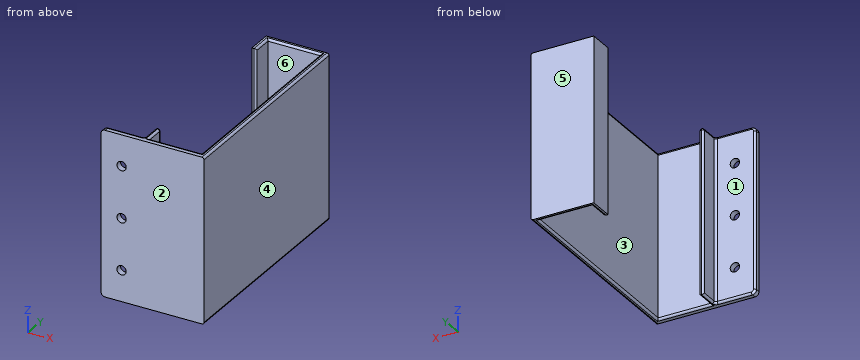
from build123d import *

# Parameters (mm, degrees)
SKETCH1_W           = 50
SKETCH1_H           = 80
BOSS_EXTRUDE1_DEPTH = 3
SKETCH2_R           = 2.25
CUT_EXTRUDE1_DEPTH  = 48.265209192
SKETCH3_W           = 2.8
SKETCH3_H           = 80
SKETCH3_W_2         = 2
BOSS_EXTRUDE2_DEPTH = 10
SKETCH4_W           = 2.8
SKETCH4_H           = 80
BOSS_EXTRUDE3_DEPTH = 90.2
SKETCH5_W           = 30.5
SKETCH5_H           = 80
BOSS_EXTRUDE4_DEPTH = 2
SKETCH6_W           = 2
SKETCH6_H           = 80
BOSS_EXTRUDE5_DEPTH = 10
FILLET1_R           = 1
FILLET2_R           = 2


# Some blends are built 0.0001 mm under size
with BuildPart() as part:
    # Sketch1 → Boss-Extrude1 (new body)
    with BuildSketch(Plane(origin=(0, 0, 0), x_dir=(1, 0, 0), z_dir=(0, 1, 0))):
        Rectangle(SKETCH1_W, SKETCH1_H)
    extrude(amount=BOSS_EXTRUDE1_DEPTH)

    # Sketch2 → Cut-Extrude1 (cut, through all)
    with BuildSketch(Plane(origin=(0, 3, 0), x_dir=(1, 0, 0), z_dir=(0, 1, 0))):
        with Locations(Location((-15, 0, 0), (0, 0, 270))):
            Circle(SKETCH2_R)
        with Locations(Location((-15, 25, 0), (0, 0, 270))):
            Circle(SKETCH2_R)
        with Locations(Location((-15, -25, 0), (0, 0, 270))):
            Circle(SKETCH2_R)
    extrude(amount=-CUT_EXTRUDE1_DEPTH, mode=Mode.SUBTRACT)

    # Sketch3 → Boss-Extrude2 (add)
    with BuildSketch(Plane(origin=(0, 3, 0), x_dir=(1, 0, 0), z_dir=(0, 1, 0))):
        with Locations((23.6, 0)):
            Rectangle(SKETCH3_W, SKETCH3_H)
        with Locations((-4.5, 0)):
            Rectangle(SKETCH3_W_2, SKETCH3_H)
    extrude(amount=BOSS_EXTRUDE2_DEPTH)

    # Sketch4 → Boss-Extrude3 (add)
    with BuildSketch(Plane(origin=(0, 13, 0), x_dir=(1, 0, 0), z_dir=(0, 1, 0))):
        with Locations((23.6, 0)):
            Rectangle(SKETCH4_W, SKETCH4_H)
    extrude(amount=BOSS_EXTRUDE3_DEPTH)

    # Sketch5 → Boss-Extrude4 (add)
    with BuildSketch(Plane(origin=(0, 103.2, 0), x_dir=(1, 0, 0), z_dir=(0, 1, 0))):
        with Locations((9.75, 0)):
            Rectangle(SKETCH5_W, SKETCH5_H)
    extrude(amount=BOSS_EXTRUDE4_DEPTH)

    # Sketch6 → Boss-Extrude5 (add)
    with BuildSketch(Plane.XZ.offset(-103.2)):
        with Locations((-4.5, 0)):
            Rectangle(SKETCH6_W, SKETCH6_H)
    extrude(amount=BOSS_EXTRUDE5_DEPTH)

    # Fillet1
    fillet1_edges = [part.edges().sort_by_distance(p)[0] for p in [
        (-25, 3, 0),
        (-15.25, 3, 40),
        (9.35, 3, -40),
        (22.2, 53.1, 40),
        (22.2, 53.1, -40),
        (-15.25, 3, -40),
        (9.35, 3, 40),
        (-5.5, 8, 40),
        (-3.5, 8, 40),
        (-3.5, 8, -40),
        (-5.5, 3, 0),
        (-5.5, 8, -40),
        (-4.5, 13, 40),
        (-3.5, 13, 0),
        (-5.5, 13, 0),
        (9.35, 103.2, -40),
        (25, 52.6, 40),
        (25, 52.6, -40),
        (9.35, 103.2, 40),
        (-3.5, 98.2, -40),
        (-3.5, 98.2, 40),
        (-3.5, 93.2, 0),
    ]]
    fillet(fillet1_edges, radius=FILLET1_R - 0.0001)  # a hair under: the kernel refuses the full size

    # Fillet2
    # the kernel refuses this fillet: 2 mm, written as the material it takes off along each edge
    with BuildSketch(Plane(origin=(-23, 3, 38), x_dir=(-1, 0, 0), z_dir=(0, 0, -1))) as fillet2_piece_1:
        with BuildLine():
            CenterArc((1.0001, -0.9999), 0.9999, 0, 90)
            Line((2, -0.9999), (2, 0))
            Line((2, 0), (1.0001, 0))
        make_face()
    revolve(axis=Axis((-23, 3, 38), (0, 1, 0)), revolution_arc=90, mode=Mode.SUBTRACT)
    with BuildSketch(Plane(origin=(-23, 3, -38), x_dir=(0, 0, -1), z_dir=(1, 0, 0))) as fillet2_piece_2:
        with BuildLine():
            CenterArc((1.0001, -0.9999), 0.9999, 0, 90)
            Line((2, -0.9999), (2, 0))
            Line((2, 0), (1.0001, 0))
        make_face()
    revolve(axis=Axis((-23, 3, -38), (0, 1, 0)), revolution_arc=90, mode=Mode.SUBTRACT)
    with BuildSketch(Plane(origin=(-25, -5, 40), x_dir=(0, 0, -1), z_dir=(0, 1, 0)), Plane(origin=(-25, -5, -40), x_dir=(1, 0, 0), z_dir=(0, 1, 0))) as fillet2_piece_3:
        with BuildLine():
            CenterArc((FILLET2_R, -FILLET2_R), FILLET2_R, 90, 90)
            Line((0, -FILLET2_R), (0, 0))
            Line((0, 0), (FILLET2_R, 0))
        make_face()
    extrude(amount=8, mode=Mode.SUBTRACT)


solid = part.part
Geometry: final body of the model. Coordinates: model frame, mm. Face numbers are marked on the shaded views. A direction names the side the tool comes from. Give positions to 0.01 mm unless a question says otherwise; leave off trailing zeros. Order: outer loops, then holes, each group sorted by start corner. A loop starts at its lowest first (then second) coordinate and runs counter-clockwise, first axis right, second up. Notation, with made-up numbers: (33.5, 59.25) -> (83.5, 59.25) arc R17 ccw to (83.5, 80.25) -> close; hole circle Ø11 at (-16.5, 39.5). An arc over 180 degrees is marked (long way). Put each result on its own line as item: value.
Q1. Pin query (flat end, axial travel): pin 1 (2 mm diameter, centred on y = 66, z = 6, fed in from -X); pin 2 (9.5 mm diameter, centred on y = 96.5, z = 6.5, fed in from -X); pin 3 (10 mm diameter, centred on x = 7.5, z = -4, fed in from -Y); pin 4 (5.5 mm diameter, centred on x = -15.5, z = 0, fed in from +Y). Return the tip coordinate at first contact, or that it passes through.
Here are the results:
pin 1: stops at x = 22.2
pin 2: stops at x = -5.5
pin 3: stops at y = 0
pin 4: stops at y = 3
Q2. Draft query along Y for the marked faces 4, 5 and 6. Return one class per face: released by +Y, released by -Y, zero draft, split by the parting line, or undercut.
Here are the results:
face 4: zero draft
face 5: released by +Y
face 6: undercut
Q3. Material intervals for L1, parallel to Y at x = 12, z = -20.5; L2, parallel to X at y = 1.5, z = 25; L3, parallel to X at y = 63, z = 15.5, sorted ascending.
Here are the results:
L1: y = 0 to 3, 103.2 to 105.2
L2: x = -25 to -17.25, -12.75 to 25
L3: x = 22.2 to 25
Q4. Reachability of the marked faces 1, 2 and 3 from +Z, -Z, +X, -X, +Y, -Y: full face, straight path, thin tool, end or side. Return the list, or none.
Here are the results:
face 1: +Z, -Z, -X, +Y
face 2: +Z, -Z, +X, -X, -Y
face 3: +Z, -Z
Q5. Section B-B, the plane x = -15. Return loops of the section in (y, z).
Here are the results:
outline: (0, -40) -> (2, -40) arc R1 ccw to (3, -39) -> (3, -27.25) -> (0, -27.25) -> close; (0, -22.75) -> (3, -22.75) -> (3, -2.25) -> (0, -2.25) -> close; (0, 2.25) -> (3, 2.25) -> (3, 22.75) -> (0, 22.75) -> close; (0, 27.25) -> (3, 27.25) -> (3, 39) arc R1 ccw to (2, 40) -> (0, 40) -> close
Q6. Section D-D, the plane y = 75. Return loops of the section in (x, z).
Here are the results:
outline: (22.2, -39) arc R1 ccw to (23.2, -40) -> (24, -40) arc R1 ccw to (25, -39) -> (25, 39) arc R1 ccw to (24, 40) -> (23.2, 40) arc R1 ccw to (22.2, 39) -> close
Q7. Section A-A, the plane x = 16.5. Return loops of the section in (y, z).
Here are the results:
outline: (0, -40) -> (2, -40) arc R1 ccw to (3, -39) -> (3, 39) arc R1 ccw to (2, 40) -> (0, 40) -> close; (103.2, -39) arc R1 ccw to (104.2, -40) -> (105.2, -40) -> (105.2, 40) -> (104.2, 40) arc R1 ccw to (103.2, 39) -> close
